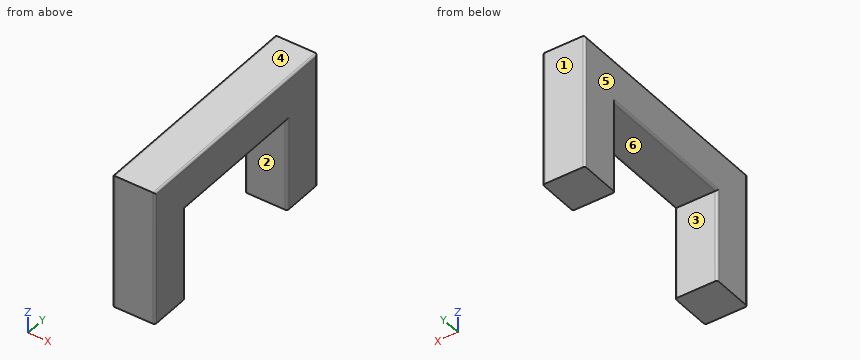
from build123d import *

# Parameters (mm, degrees)
F1_DEPTH = 100
F2_R     = 5


with BuildPart() as f1:
    # F0 (on Right) → F1 (new body)
    with BuildSketch(Plane.YZ):
        Polygon((0, 220), (0, 0), (100, 0), (100, 320), (-440, 320), (-440, 0), (-340, 0), (-340, 220), align=None)
    extrude(amount=F1_DEPTH)

    # F2
    f2_edges = [f1.edges().sort_by_distance(p)[0] for p in [
        (100, -440, 160),
        (100, -340, 110),
        (100, -170, 220),
        (100, 0, 110),
        (100, 100, 160),
        (0, -440, 160),
        (0, 0, 110),
        (0, -170, 220),
        (0, -340, 110),
        (0, 100, 160),
        (0, -170, 320),
        (100, -170, 320),
    ]]
    fillet(f2_edges, radius=F2_R)


solid = f1.part
The model under review builds one solid part; all positions refer to its coordinate system, in mm. Face numbers are marked on the shaded views. A direction names the side the tool comes from. Coordinates: 2 decimals unless noted, no trailing zeros. Order: outer loops, then holes, each group sorted by start corner. A loop starts at its lowest first (then second) coordinate and runs counter-clockwise, first axis right, second up. Notation, with made-up numbers: (36.5, -25.75) -> (92.5, -25.75) arc R14 cw to (92.5, -0.75) -> close; hole circle Ø11 at (22.25, 4.5). An arc over 180 degrees is marked (long way). Answer in a Markdown table with one row per item.
(1) Insertion check: pin 1 (12 mm diameter, centred on y = -225, z = 212.5, fed in from +X); pin 2 (1.5 mm diameter, centred on y = 0.5, z = 50, fed in from -X); pin 3 (1 mm diameter, centred on x = 86, y = -13, fed in from -Z). Each pin has a flat end and moves straight along its axis. Give the tip position at first contact, or say it passes through.
Answers:
| item | result |
|---|---|
| pin 1 | through |
| pin 2 | x = 1.69 |
| pin 3 | z = 220 |
(2) Consider section A-A (z = 101). Write out the cut boundary in (x, y), plus the area to 3 significant figures.
Answers:
| item | result |
|---|---|
| outline | (0, -435) arc R5 ccw to (5, -440) -> (95, -440) arc R5 ccw to (100, -435) -> (100, -345) arc R5 ccw to (95, -340) -> (5, -340) arc R5 ccw to (0, -345) -> close; (0, 5) arc R5 ccw to (5, 0) -> (95, 0) arc R5 ccw to (100, 5) -> (100, 95) arc R5 ccw to (95, 100) -> (5, 100) arc R5 ccw to (0, 95) -> close |
| area | 20,000 mm² |
(3) Consider section C-C (x = 59.5). Write out the cut boundary in (y, z), plus the area to 3 significant figures.
Answers:
| item | result |
|---|---|
| outline | (-440, 0) -> (-340, 0) -> (-340, 220) -> (0, 220) -> (0, 0) -> (100, 0) -> (100, 320) -> (-440, 320) -> close |
| area | 98,000 mm² |
(4) Wall thickness on line 1 along Y through (x, z) = (67, 198.5); line 2 along Z through (x, y) = (12, -104.5): over which ranges is each line inside the solid? List them lowest first.
Answers:
| item | result |
|---|---|
| line 1 | -440 to -340, 0 to 100 |
| line 2 | 220 to 320 |
(5) The part is to be moulded in two halves that separate along Y. For the marked faces 1, 2, 3 and 4, say which applies: +Y half, -Y half, draft (parallel to the pull), parting line (faces both ways), or undercut.
Answers:
| item | result |
|---|---|
| face 1 | +Y half |
| face 2 | undercut |
| face 3 | undercut |
| face 4 | draft |
(6) Consider section B-B (y = -173). Write out the cut boundary in (x, z).
Answers:
| item | result |
|---|---|
| outline | (0, 225) arc R5 ccw to (5, 220) -> (95, 220) arc R5 ccw to (100, 225) -> (100, 315) arc R5 ccw to (95, 320) -> (5, 320) arc R5 ccw to (0, 315) -> close |
(7) Machinability: for the marked faces 5 and 6, which of the approach directions +Z, -Z, +X, -X, +Y, -Y give a long, thin tool a straight path to every point of the face, cutting with its end or side? Answer none if there is none.
Answers:
| item | result |
|---|---|
| face 5 | +Z, -Z, -X, +Y, -Y |
| face 6 | -Z, +X, -X |
